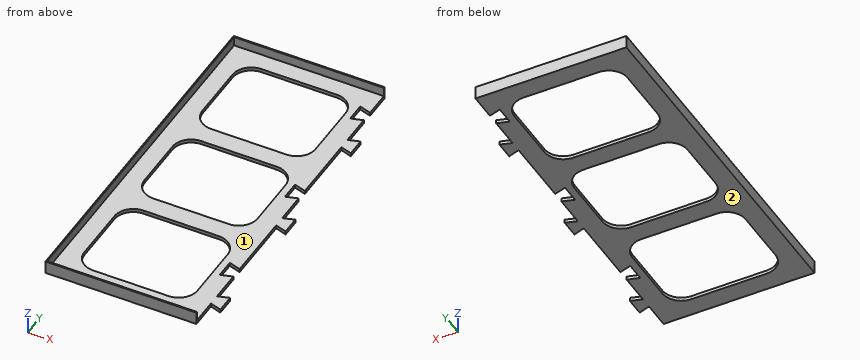
```python
from build123d import *

# Parameters (mm, degrees)
F1_DEPTH = 1.5
F2_W     = 48
F2_H     = 39.9
F2_H_2   = 38.2
F3_DEPTH = 1.501
F4_R     = 8
F6_DEPTH = 4


with BuildPart() as f1:
    # F0 (on Top) → F1 (new body)
    with BuildSketch(Plane.XY):
        Polygon((0, 150), (0, 0), (64, 0), (64, 11.6), (68.8, 10.1), (68.8, 17.9), (64, 16.4), (64, 29.5), (59, 28), (59, 36), (64, 34.5), (64, 63.6), (68.8, 62.1), (68.8, 69.9), (64, 68.4), (64, 81.5), (59, 80), (59, 88), (64, 86.5), (64, 115.6), (68.8, 114.1), (68.8, 121.9), (64, 120.4), (64, 133.5), (59, 132), (59, 140), (64, 138.5), (64, 150), align=None)
    extrude(amount=F1_DEPTH)

    # F2 (on face) → F3 (cut, through all)
    with BuildSketch(Plane.XY.offset(1.5)):
        with Locations((32, 122.05)):
            Rectangle(F2_W, F2_H)
        with Locations((32, 75)):
            Rectangle(F2_W, F2_H_2)
        with Locations((32, 27.95)):
            Rectangle(F2_W, F2_H)
    extrude(amount=-F3_DEPTH, mode=Mode.SUBTRACT)

    # F4
    f4_edges = [f1.edges().sort_by_distance(p)[0] for p in [
        (8, 142, 0.75),
        (8, 94.1, 0.75),
        (8, 47.9, 0.75),
        (56, 142, 0.75),
        (56, 94.1, 0.75),
        (56, 47.9, 0.75),
        (56, 102.1, 0.75),
        (56, 55.9, 0.75),
        (56, 8, 0.75),
        (8, 8, 0.75),
        (8, 55.9, 0.75),
        (8, 102.1, 0.75),
    ]]
    fillet(f4_edges, radius=F4_R)

    # F5 (on face) → F6 (join)
    with BuildSketch(Plane.XY.offset(1.5)):
        Polygon((64, 149.5), (64, 150), (0, 150), (0, 0), (64, 0), (64, 0.5), (0.5, 0.5), (0.5, 149.5), align=None)
    extrude(amount=F6_DEPTH)


solid = f1.part
```
Design review of the part built by this model. Coordinates are the model's own, in mm. Face numbers are marked on the shaded views. Coordinates: 2 decimals unless noted, no trailing zeros. Loops run counter-clockwise (first coordinate to the right, second up) from the corner with the lowest first, then second, coordinate; pieces in that order, holes last. Notation, with made-up numbers: M 28.5,87.25 L 76.5,87.25 A22 ccw 76.5,98.25 Z; hole C 9,-33.5 d4. An arc over 180 degrees is marked long. One line per question, with ' | ' between items.
(1) We need section A-A (x = 37). Give the boundary of the cut face in (y, z), and give its area (3 significant figures).
Filled in:
outline: M 0,0 L 8,0 L 8,1.5 L 0.5,1.5 L 0.5,5.5 L 0,5.5 Z; M 47.9,0 L 55.9,0 L 55.9,1.5 L 47.9,1.5 Z; M 94.1,0 L 102.1,0 L 102.1,1.5 L 94.1,1.5 Z; M 142,0 L 150,0 L 150,5.5 L 149.5,5.5 L 149.5,1.5 L 142,1.5 Z | area: 52.0 mm^2
(2) Wall thickness on probe 1 along Y at (x, z) = (19.5, 4.75); probe 2 along Y at (x, z) = (17.5, 0.85); probe 3 along X at (y, z) = (59, 3.2): over which ranges is each line inside the solid? List them lowest first.
Filled in:
probe 1: y = 0 to 0.5, 149.5 to 150 | probe 2: y = 0 to 8, 47.9 to 55.9, 94.1 to 102.1, 142 to 150 | probe 3: x = 0 to 0.5
(3) We need section C-C (z = 3.2). Give the boundary of the cut face in (x, y).
Filled in:
outline: M 0,0 L 64,0 L 64,0.5 L 0.5,0.5 L 0.5,149.5 L 64,149.5 L 64,150 L 0,150 Z
(4) For pin 1 Ø1.6 at (y, z) = (53.5, 1) entering from +X; pin 2 Ø1.6 at (y, z) = (135, 0.5) entering from +X; pin 3 Ø6 at (x, y) = (51.5, 24.5) entering from +Z; pin 4 Ø1.5 at (x, y) = (25, 49) entering from +Z, all flat-tipped, find the tip position at first contact; note any pin that passes through.
Filled in:
pin 1: stops at x = 64 | pin 2: stops at x = 59 | pin 3: passes through | pin 4: stops at z = 1.5
(5) Draft analysis for pull direction Y (two halves, no side actions). For the marked faces 1 and 2, state which applies: released by +Y, released by -Y, zero draft, split by the parting line, or undercut.
Filled in:
face 1: undercut | face 2: zero draft
(6) We need section B-B (y = 111.5). Give the boundary of the cut face in (x, z), and give its area (3 significant figures).
Filled in:
outline: M 0,0 L 8,0 L 8,1.5 L 0.5,1.5 L 0.5,5.5 L 0,5.5 Z; M 56,0 L 64,0 L 64,1.5 L 56,1.5 Z | area: 26.0 mm^2
(7) We need section D-D (x = 5). Give the boundary of the cut face in (y, z).
Filled in:
outline: M 0,0 L 150,0 L 150,5.5 L 149.5,5.5 L 149.5,1.5 L 0.5,1.5 L 0.5,5.5 L 0,5.5 Z
